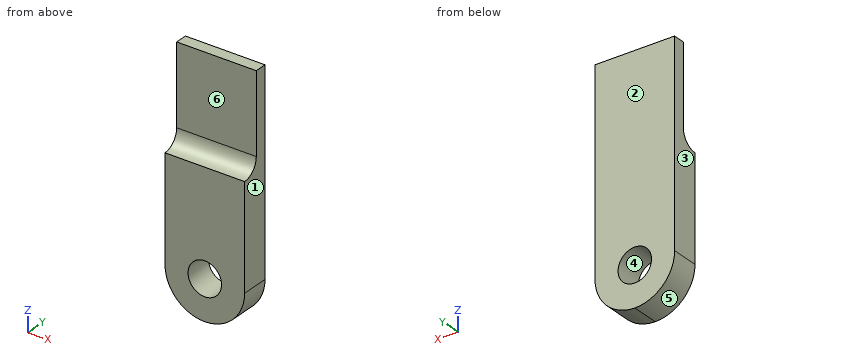
```python
from build123d import *

# Parameters (mm, degrees)
CROQUIS1_W              = 10
CROQUIS1_H              = 30
SALIENTE_EXTRUIR1_DEPTH = 1.75
REDONDEO1_R             = 5
CROQUIS2_R              = 2.1
CORTAR_EXTRUIR1_DEPTH   = 3.5
CROQUIS3_W              = 10
CROQUIS3_H              = 12
CORTAR_EXTRUIR2_DEPTH   = 2
REDONDEO2_R             = 2


with BuildPart() as part:
    # Croquis1 → Saliente-Extruir1 (new, symmetric)
    with BuildSketch(Plane(origin=(0, 0, 0), x_dir=(1, 0, 0), z_dir=(0, 1, 0))):
        Rectangle(CROQUIS1_W, CROQUIS1_H)
    extrude(amount=SALIENTE_EXTRUIR1_DEPTH, both=True)

    # Redondeo1
    redondeo1_edges = [part.edges().sort_by_distance(p)[0] for p in [
        (5, 0, -15),
        (-5, 0, -15),
    ]]
    fillet(redondeo1_edges, radius=REDONDEO1_R - 0.0001)  # a hair under: the kernel refuses the full size

    # Croquis2 → Cortar-Extruir1 (cut)
    with BuildSketch(Plane(origin=(0, 1.75, 0), x_dir=(1, 0, 0), z_dir=(0, 1, 0))):
        with Locations(Location((0, 10, 0), (0, 0, 270))):
            Circle(CROQUIS2_R)
    extrude(amount=-CORTAR_EXTRUIR1_DEPTH, mode=Mode.SUBTRACT)

    # Croquis3 → Cortar-Extruir2 (cut)
    with BuildSketch(Plane.XZ.offset(1.75)):
        with Locations((0, 9)):
            Rectangle(CROQUIS3_W, CROQUIS3_H)
    extrude(amount=-CORTAR_EXTRUIR2_DEPTH, mode=Mode.SUBTRACT)

    # Redondeo2
    redondeo2_edges = [part.edges().sort_by_distance(p)[0] for p in [
        (0, 0.25, 3),
    ]]
    fillet(redondeo2_edges, radius=REDONDEO2_R - 0.0001)  # a hair under: the kernel refuses the full size


solid = part.part
```
Here's how the part is built. I have some questions about the finished solid (model axes, mm). Face numbers are marked on the shaded views. A direction names the side the tool comes from. Coordinates: 2 decimals unless noted, no trailing zeros. Order: outer loops, then holes, each group sorted by start corner. A loop starts at its lowest first (then second) coordinate and runs counter-clockwise, first axis right, second up. Notation, with made-up numbers: (-22.75, 42.5) - (-18.75, 42.5) arc R37 ccw to (-18.75, 78.5) - close; hole circle Ø6 at (57, -4). An arc over 180 degrees is marked (long way). One line per question, with ' | ' between items. Start each with the question number.
1. Please list where these lines run through material, in increasing order: line 1 along X through (y, z) = (-0.35, -10); line 2 along X through (y, z) = (-1.55, -8.75); line 3 along Y through (x, z) = (-4.25, 12.5). Write a range as [from, to].
2. If we section it at A-A (z = -10.75): Write out the boundary of the cut face in (x, y).
3. I'm going to push flat-ended pins straight in: pin 1 Ø2 at (x, y) = (-4, 0.5) entering from -Z; pin 2 Ø1.5 at (x, y) = (-1.5, -1) entering from -Z. Where does each tip first touch, or does it pass through?
4. If we mould it in two halves opening along X, with no side actions, what happens to the marked faces 1, 2, 3 and 4? For each: released by +X, released by -X, zero draft, split by the parting line, or undercut.
5. Which directions (+Z, -Z, +X, -X, +Y, -Y) give clear straight access to the entire face, cutting with the end or side of a thin tool? Please do the marked faces 5 and 6.
6. If we section it at D-D (z = 10.5): Write out the boundary of the cut face in (x, y).
Model answer:
1) line 1: x = [-5, -2.1], [2.1, 5] | line 2: x = [-5, -1.69], [1.69, 5] | line 3: y = [0.25, 1.75]
2) outline: (-4.94, -1.75) - (-1.96, -1.75) - (-1.96, 1.75) - (-4.94, 1.75) - close; (1.96, -1.75) - (4.94, -1.75) - (4.94, 1.75) - (1.96, 1.75) - close
3) pin 1: stops at z = -14 | pin 2: stops at z = -14.94
4) face 1: released by +X | face 2: zero draft | face 3: released by -X | face 4: undercut
5) face 5: -Z, -X, +Y, -Y | face 6: +Z, +X, -X, -Y
6) outline: (-5, 0.25) - (5, 0.25) - (5, 1.75) - (-5, 1.75) - close
